Autodesk Inventor part; units mm, degrees
ref_plane "YZ Plane" through (0, 0, 0) normal (1, 0, 0) x (0, 1, 0)
ref_plane "XZ Plane" through (0, 0, 0) normal (0, 1, 0) x (-1, 0, 0)
ref_plane "XY Plane" through (0, 0, 0) normal (0, 0, 1) x (1, 0, 0)
sketch "Sketch1" plane through (0, 0, 0) normal (0, 0, 1) x (1, 0, 0)
  line L0 (-50, -50) -> (50, -50)
  line L1 (50, -50) -> (50, 50)
  line L2 (50, 50) -> (-50, 50)
  line L3 (-50, 50) -> (-50, -50)
  line L4 (-50, -50) -> (50, 50) construction
  line L5 (50, -50) -> (-50, 50) construction
  point P0 (0, 0)
  dimension "d0" = 100
  dimension "d1" = 100
extrude "Extrusion1" add sketch "Sketch1" along normal blind 5
sketch "Sketch2" plane through (-50, 50, 0) normal (0, 1, 0) x (1, 0, 0)
  line L0 (0, 0) -> (100, 0)
  line L1 (0, 0) -> (49.9986, 49.9986)
  line L2 (49.9986, 49.9986) -> (53.5341, 46.463)
  line L3 (53.5341, 46.463) -> (3.5355, -3.5355)
  line L4 (3.5355, -3.5355) -> (0, 0)
  line L5 (0, 0) -> (70.7086, 0) construction
  line L6 (100.108, -0.1109) -> (53.5341, 46.463)
  line L7 (53.5341, 46.463) -> (49.9986, 42.9275)
  line L8 (49.9986, 42.9275) -> (96.5724, -3.6464)
  line L9 (96.5724, -3.6464) -> (100.108, -0.1109)
  point P0 (50, 0)
  point P1 (49.9986, 42.9275)
  dimension "d4" = 45
  dimension "d5" = 5
  dimension "d6" = 5
extrude "Extrusion2" add sketch "Sketch2" against normal blind 55 contours L1 L2 L3 L0 | L0 L3 L4 | L8 L3 L6 L0 | L0 L6 L9 L8
sketch "Sketch3" plane through (0, 0, 5) normal (0, 0, 1) x (1, 0, 0)
  line L0 (2.5, -25) -> (-2.5, -25)
  line L1 (-17.5, -10) -> (-17.5, 10)
  line L2 (-2.5, 25) -> (2.5, 25)
  line L3 (17.5, 10) -> (17.5, -10)
  line L4 (17.5, -25) -> (-17.5, 25) construction
  line L5 (-17.5, -25) -> (17.5, 25) construction
  arc A0 (-2.5, 25) -> (-17.5, 10) centre (-2.5, 10) ccw
  arc A1 (17.5, 10) -> (2.5, 25) centre (2.5, 10) ccw
  arc A2 (2.5, -25) -> (17.5, -10) centre (2.5, -10) ccw
  arc A3 (-17.5, -10) -> (-2.5, -25) centre (-2.5, -10) ccw
  point P0 (0, 0)
  dimension "d9" = 35
  dimension "d10" = 50
  dimension "d11" = 15
extrude "Extrusion3" cut sketch "Sketch3" against normal blind 5
properties part number "fixation_v03"
Can you work these out from the model? Positions are in its coordinate system, mm. A direction names the side the tool comes from. Coordinates: 2 decimals unless noted, no trailing zeros. Loops run counter-clockwise (first coordinate to the right, second up) from the corner with the lowest first, then second, coordinate; pieces in that order, holes last.
Item 1: Suppose I cut it at A-A (y = -7). Please give me the cut outline in (x, z), then the cut area to 3 significant figures.
Answers below:
outline: (-50, 0) - (-17.5, 0) - (-17.5, 5) - (-50, 5) - close; (17.5, 0) - (50, 0) - (50, 5) - (17.5, 5) - close
area: 325 mm2
Item 2: If we mould it in two halves opening along Y, with no side actions, what happens to faces 4 (the face through (12.99, -20.72, 2.54)), 5 (the face through (0, 50, 2)), 6 (the face through (22, 1, 0))? For each: released by +Y, released by -Y, zero draft, split by the parting line, or undercut.
Answers below:
face 4: undercut
face 5: released by +Y
face 6: zero draft
Item 3: Please list where these lines run through material, in increasing order: L1, parallel to X at y = 40.5, z = -11; L2, parallel to Z at x = 35, y = 27; L3, parallel to Z at x = -1.5, y = -36.5.
Answers below:
L1: x = -39 to -31.93, 31.93 to 39
L2: z = -15 to -7.93, 0 to 5
L3: z = 0 to 5
Item 4: Suppose I cut it at B-B (x = -13.5). Please give me the cut outline in (y, z), then the cut area to 3 significant figures.
Answers below:
outline: (-50, 0) - (-20.2, 0) - (-20.2, 5) - (-50, 5) - close; (-5, -36.5) - (50, -36.5) - (50, -29.43) - (-5, -29.43) - close; (20.2, 0) - (50, 0) - (50, 5) - (20.2, 5) - close
area: 687 mm2
Item 5: Suppose I cut it at C-C (z = -3). Please give me the cut outline in (x, y), then the cut area to 3 significant figures.
Answers below:
outline: (-47, -5) - (-39.93, -5) - (-39.93, 50) - (-47, 50) - close; (39.93, -5) - (47, -5) - (47, 50) - (39.93, 50) - close
area: 778 mm2
Item 6: Which directions (+Z, -Z, +X, -X, +Y, -Y) give clear straight access to the entire face, cutting with the end or side of a thin tool? Please do faces 1 (the face through (-17.5, 0, 3)), 2 (the face through (-21.165, 22.885, -21.764)), 3 (the face through (0, -25, 3)).
Answers below:
face 1: +Z
face 2: +Y, -Y
face 3: +Z, -Z
Item 7: I'm going to push flat-ended pins straight in: pin 1 (5 mm diameter, centred on y = 3, z = -18.5, fed in from +X); pin 2 (3 mm diameter, centred on y = 24.5, z = -18, fed in from -X); pin 3 (4 mm diameter, centred on y = -18, z = 3.5, fed in from +X). Where does each tip first touch, or does it pass through?
Answers below:
pin 1: stops at x = 34
pin 2: stops at x = -33.5
pin 3: stops at x = 50
